```python
from build123d import *

# Parameters (mm, degrees)
F0_R     = 5
F0_R_2   = 4.1
F1_DEPTH = 2
F2_SIZE  = 0.2
F3_W     = 1
F3_H     = 0.5
F4_DEPTH = 25


with BuildPart() as f1:
    # F0 (on Top) → F1 (new body)
    with BuildSketch(Plane.XY):
        Circle(F0_R)
        Circle(F0_R_2, mode=Mode.SUBTRACT)
    extrude(amount=F1_DEPTH)

    # F2
    f2_edges = [f1.edges().sort_by_distance(p)[0] for p in [
        (-5, 0, 2),
    ]]
    chamfer(f2_edges, length=F2_SIZE)


with BuildPart() as f4:
    # F3 (on Front) → F4 (new body)
    with BuildSketch(Plane.XZ):
        with Locations((0.5, 1.840964)):
            Rectangle(F3_W, F3_H)
    extrude(amount=F4_DEPTH)


with BuildPart() as f4_1:
    # F5: moved
    add(f4.part.moved(Location((-0.5, 13.3, 0))))


with BuildPart() as f1_1:
    add(f1.part)

    # F6: cut F4
    add(f4_1.part, mode=Mode.SUBTRACT)


solid = f1_1.part
```
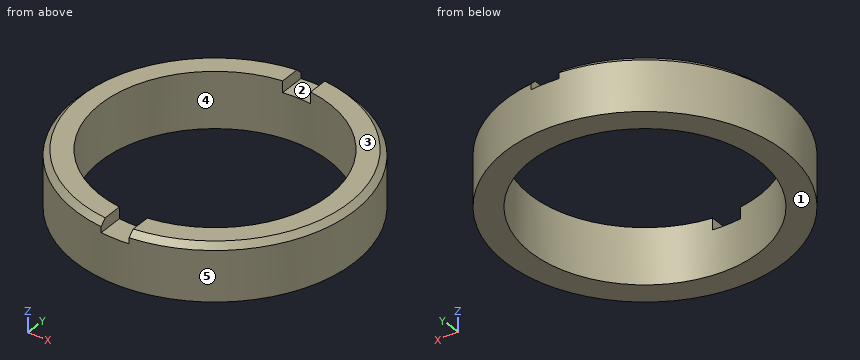
Here's how the part is built. I have some questions about the finished solid (model axes, mm). Face numbers are marked on the shaded views. A direction names the side the tool comes from. Give positions to 0.01 mm unless a question says otherwise; leave off trailing zeros. Loops run counter-clockwise (first coordinate to the right, second up) from the corner with the lowest first, then second, coordinate; pieces in that order, holes last. Notation, with made-up numbers: (46, 10.5) -> (53, 10.5) arc R23 ccw to (53, 28.5) -> close; hole circle Ø6 at (-2, 42). An arc over 180 degrees is marked (long way). Use one line per item in the form item = value. Start each with the question number.
1) Which directions (+Z, -Z, +X, -X, +Y, -Y) give clear straight access to the entire face, cutting with the end or side of a thin tool? Please do the marked faces 1 and 2.
2) For P1, Ø0.7, axis at x = 0, y = -4.5, coming from the +Z side, with a flat end and sliding along its axis, tell me the tip position at first contact or that it passes through.
3) Please list where these lines run through material, in increasing order: line 1 along X through (y, z) = (0, 0.85); line 2 along Y through (x, z) = (-1.75, 1.2).
4) Thinking about a two-plate mould opening in X: for the marked faces 3, 4 and 5, which applies, +X half, -X half, draft (parallel to the pull), parting line (faces both ways), or undercut?
5) Imagine slicing it at A-A (x = 0). Please give me the cut outline in (y, z).
6) Imagine slicing it at C-C (z = 0.25). Please give me the cut outline in (x, y).
7) Imagine slicing it at B-B (y = 0). Please give me the cut outline in (x, z).
Check values:
q1.face_1 = -Z, +X, -X, +Y, -Y
q1.face_2 = +Z, +Y, -Y
q2.P1 = 1.59
q3.line_1 = -5 to -4.1, 4.1 to 5
q3.line_2 = -4.68 to -3.71, 3.71 to 4.68
q4.face_3 = draft
q4.face_4 = undercut
q4.face_5 = parting line
q5.outline = (-5, 0) -> (-4.1, 0) -> (-4.1, 1.59) -> (-5, 1.59) -> close; (4.1, 0) -> (5, 0) -> (5, 1.59) -> (4.1, 1.59) -> close
q6.outline = circle Ø10 at (0, 0); hole circle Ø8.2 at (0, 0)
q7.outline = (-5, 0) -> (-4.1, 0) -> (-4.1, 2) -> (-4.8, 2) -> (-5, 1.8) -> close; (4.1, 0) -> (5, 0) -> (5, 1.8) -> (4.8, 2) -> (4.1, 2) -> close
